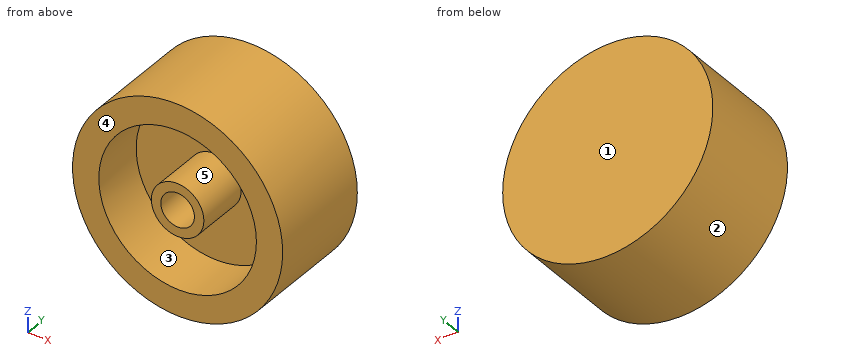
from build123d import *

# Parameters (mm, degrees)
F0_R     = 12.7
F1_DEPTH = 12.7
F2_R     = 9.525
F3_DEPTH = 6.35
F4_R     = 3.175
F5_DEPTH = 6.35
F6_R     = 2.032
F7_DEPTH = 6.35


with BuildPart() as f1:
    # F0 (on Front) → F1 (new body)
    with BuildSketch(Plane.XZ):
        Circle(F0_R)
    extrude(amount=F1_DEPTH)

    # F2 (on face) → F3 (cut)
    with BuildSketch(Plane.XZ.offset(12.7)):
        Circle(F2_R)
    extrude(amount=-F3_DEPTH, mode=Mode.SUBTRACT)

    # F4 (on face) → F5 (join, through all)
    with BuildSketch(Plane.XZ.offset(6.35)):
        Circle(F4_R)
    extrude(amount=F5_DEPTH)

    # F6 (on face) → F7 (cut, through all)
    with BuildSketch(Plane.XZ.offset(12.7)):
        Circle(F6_R)
    extrude(amount=-F7_DEPTH, mode=Mode.SUBTRACT)


solid = f1.part
The model under review builds one solid part; all positions refer to its coordinate system, in mm. Face numbers are marked on the shaded views. A direction names the side the tool comes from. Round coordinates to 2 decimals unless told otherwise and drop trailing zeros. Loops run counter-clockwise (first coordinate to the right, second up) from the corner with the lowest first, then second, coordinate; pieces in that order, holes last. Notation, with made-up numbers: M 48.25,8 L 60.25,8 A18 cw 60.25,26 Z; hole C 32.25,43.25 d7. An arc over 180 degrees is marked long. Answer as CSV lines item,"result". Start each with the question number.
Item 1: Consider section B-B (x = 0). Write out the cut boundary in (y, z) (3 decimals), then the cut area to 3 significant figures.
Item 2: Consider section C-C (z = -6). Write out the cut boundary in (x, y).
Item 3: For the marked faces 4 and 5, list the 3-axis set-ups (+Z, -Z, +X, -X, +Y, -Y) from which the entire face can be reached by the end or side of a thin tool; tool diameter is ignored.
Item 4: Insertion check: P1, Ø1.5, axis at x = 4.5, z = 1, coming from the -Y side; P2, Ø6, axis at y = -10.5, z = -5, coming from the +X side; P3, Ø5, axis at y = -10.5, z = -8, coming from the +X side. Each pin has a flat end and moves straight along its axis. Give the tip position at first contact, or say it passes through.
Item 5: Wall thickness on line 1 (Z direction, x = 0, y = -8.5) (3 decimals); line 2 (Z direction, x = 1.25, y = -10); line 3 (X direction, y = -8.25, z = -2.5): over which ranges is each line inside the solid? List them lowest first. Write a range as [from, to].
Item 6: Consider section A-A (y = -7.75). Write out the cut boundary in (x, z) (3 decimals), then the cut area to 3 significant figures.
Item 7: Mouldability with a two-part tool opening along X and no side actions: class the marked faces 1, 2 and 3 as released by +X, released by -X, zero draft, split by the parting line, or undercut.
Item 8: Consider section D-D (y = -1). Write out the cut boundary in (x, z), then the cut area to 3 significant figures.
Answer:
1,outline,"M -12.7,-12.7 L 0,-12.7 L 0,12.7 L -12.7,12.7 L -12.7,9.525 L -6.35,9.525 L -6.35,3.175 L -12.7,3.175 L -12.7,2.032 L -6.35,2.032 L -6.35,-2.032 L -12.7,-2.032 L -12.7,-3.175 L -6.35,-3.175 L -6.35,-9.525 L -12.7,-9.525 Z"
1,area,"216 mm^2"
2,outline,"M -11.19,-12.7 L -7.4,-12.7 L -7.4,-6.35 L 7.4,-6.35 L 7.4,-12.7 L 11.19,-12.7 L 11.19,0 L -11.19,0 Z"
3,face 4,"+Z, -Z, +X, -X, -Y"
3,face 5,"-Y"
4,P1,"stops at y = -6.35"
4,P2,"stops at x = 12.54"
4,P3,"stops at x = 11.45"
5,line 1,"z = [-12.7, -9.525], [-3.175, -2.032], [2.032, 3.175], [9.525, 12.7]"
5,line 2,"z = [-12.64, -9.44], [-2.92, -1.6], [1.6, 2.92], [9.44, 12.64]"
5,line 3,"x = [-12.45, -9.19], [-1.96, 1.96], [9.19, 12.45]"
6,outline,"C 0,0 d25.4; C 0,0 d6.35; hole C 0,0 d19.05; hole C 0,0 d4.064"
6,area,"240 mm^2"
7,face 1,"zero draft"
7,face 2,"split by the parting line"
7,face 3,"undercut"
8,outline,"C 0,0 d25.4"
8,area,"507 mm^2"
